Design review of the part built by this model. Coordinates are the model's own, in mm. Face numbers are marked on the shaded views. A direction names the side the tool comes from. Round coordinates to 2 decimals unless told otherwise and drop trailing zeros. Order: outer loops, then holes, each group sorted by start corner. A loop starts at its lowest first (then second) coordinate and runs counter-clockwise, first axis right, second up. Notation, with made-up numbers: (66, 51.25) - (72, 51.25) arc R27 cw to (72, 67.25) - close; hole circle Ø2 at (9, 72). An arc over 180 degrees is marked (long way). Use CSV: the item, a comma, the result in double quotes. Start each with the question number.
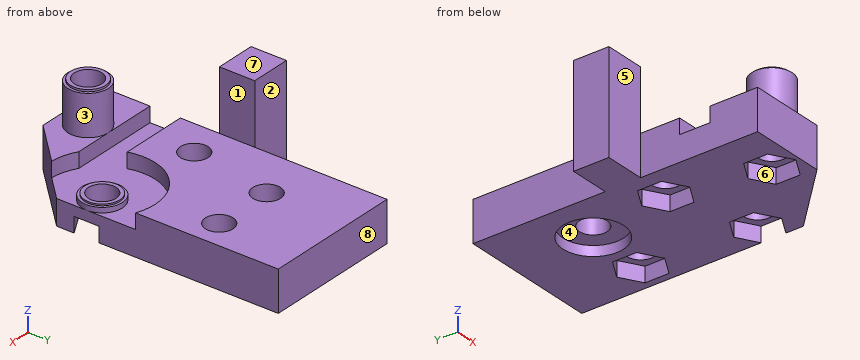
from build123d import *

# Parameters (mm, degrees)
SKETCH007_R             = 2.75
PAD004_DEPTH            = 8
POCKET003_DEPTH         = 3
SKETCH022_R             = 4
SKETCH022_R_2           = 2.75
PAD015_DEPTH            = 1
SKETCH023_R             = 3.5
SKETCH023_R_2           = 2.75
PAD016_DEPTH            = 0.3
SKETCH024_R             = 4
SKETCH024_R_2           = 2.75
PAD017_DEPTH            = 8
SKETCH025_R             = 3.5
SKETCH025_R_2           = 2.75
PAD018_DEPTH            = 0.4
SKETCH026_R             = 6
POCKET005_DEPTH         = 2
POCKET006_DEPTH         = 3
SKETCH028_W             = 7
SKETCH028_H             = 20
PAD019_DEPTH            = 8
BODY001_ROLL_ANGLE      = 180
BODY001_PLACEMENT_ANGLE = -90


with BuildPart() as part:
    # Sketch007 → Pad004 (new body)
    with BuildSketch(Plane.XY):
        Polygon((0, 27.5), (56.4, 27.5), (56.4, 12.5), (43.9, 0), (0, 0), align=None)
        with Locations((16, 17.5)):
            Circle(SKETCH007_R, mode=Mode.SUBTRACT)
        with Locations((16, 5.5)):
            Circle(SKETCH007_R, mode=Mode.SUBTRACT)
        with Locations((32.7, 20.5)):
            Circle(SKETCH007_R, mode=Mode.SUBTRACT)
        with Locations((38, 4)):
            Circle(SKETCH007_R, mode=Mode.SUBTRACT)
        with Locations((50.95, 16.95)):
            Circle(SKETCH007_R, mode=Mode.SUBTRACT)
    extrude(amount=PAD004_DEPTH)

    # Sketch012 (on Face11 of Pad004) → Pocket003 (cut)
    with BuildSketch(Plane(origin=(0, 0, 0), x_dir=(1, 0, 0), z_dir=(0, 0, -1))):
        with BuildLine():
            ThreePointArc((46.95, -9.490674), (31.623381, 4.341986), (40.95, -14.077078))
            Line((40.95, -14.077078), (40.95, -49.490674))
            Line((40.95, -49.490674), (46.95, -49.490674))
            Line((46.95, -9.490674), (46.95, -49.490674))
        make_face()
    extrude(amount=-POCKET003_DEPTH, mode=Mode.SUBTRACT)

    # Sketch022 (on Face2 of Pocket003) → Pad015 (join)
    with BuildSketch(Plane(origin=(0, 0, 3), x_dir=(1, 0, 0), z_dir=(0, 0, -1))):
        with Locations((38, -4)):
            Circle(SKETCH022_R)
        with Locations((38, -4)):
            Circle(SKETCH022_R_2, mode=Mode.SUBTRACT)
    extrude(amount=PAD015_DEPTH)

    # Sketch023 (on Face19 of Pad015) → Pad016 (join)
    with BuildSketch(Plane(origin=(0, 0, 2), x_dir=(1, 0, 0), z_dir=(0, 0, -1))):
        with Locations((38, -4)):
            Circle(SKETCH023_R)
        with Locations((38, -4)):
            Circle(SKETCH023_R_2, mode=Mode.SUBTRACT)
    extrude(amount=PAD016_DEPTH)

    # Sketch024 (on Face18 of Pad016) → Pad017 (join)
    with BuildSketch(Plane(origin=(0, 0, 0), x_dir=(1, 0, 0), z_dir=(0, 0, -1))):
        with Locations((50.95, -16.95)):
            Circle(SKETCH024_R)
        with Locations((50.95, -16.95)):
            Circle(SKETCH024_R_2, mode=Mode.SUBTRACT)
    extrude(amount=PAD017_DEPTH)

    # Sketch025 (on Face23 of Pad017) → Pad018 (join)
    with BuildSketch(Plane(origin=(0, 0, -8), x_dir=(1, 0, 0), z_dir=(0, 0, -1))):
        with Locations((50.95, -16.95)):
            Circle(SKETCH025_R)
        with Locations((50.95, -16.95)):
            Circle(SKETCH025_R_2, mode=Mode.SUBTRACT)
    extrude(amount=PAD018_DEPTH)

    # Sketch026 (on Face6 of Pad018) → Pocket005 (cut)
    with BuildSketch(Plane.XY.offset(8)):
        with Locations((16, 17.5)):
            Circle(SKETCH026_R)
    extrude(amount=-POCKET005_DEPTH, mode=Mode.SUBTRACT)

    # Sketch027 (on Face6 of Pocket005) → Pocket006 (cut)
    with BuildSketch(Plane.XY.offset(8)):
        Polygon((20.75, 5.5), (18.375, 9.613621), (13.625, 9.613621), (11.25, 5.5), (13.625, 1.386379), (18.375, 1.386379), align=None)
        Polygon((37.45, 20.5), (35.075, 24.613621), (30.325, 24.613621), (27.95, 20.5), (30.325, 16.386379), (35.075, 16.386379), align=None)
        Polygon((42.75, 4), (40.375, 8.113621), (35.625, 8.113621), (33.25, 4), (35.625, -0.113621), (40.375, -0.113621), align=None)
        Polygon((55.7, 16.95), (53.325, 21.063621), (48.575, 21.063621), (46.2, 16.95), (48.575, 12.836379), (53.325, 12.836379), align=None)
    extrude(amount=-POCKET006_DEPTH, mode=Mode.SUBTRACT)

    # Sketch028 (on Face12 of Pocket006) → Pad019 (join)
    with BuildSketch(Plane(origin=(0, 27.5, 0), x_dir=(-1, 0, 0), z_dir=(0, 1, 0))):
        with Locations((-29.7, -2)):
            Rectangle(SKETCH028_W, SKETCH028_H)
    extrude(amount=PAD019_DEPTH)


with BuildPart() as part_1:
    # Body001 roll: moved
    add(part.part.rotate(Axis((0, 0, 0), (1, 0, 0)), BODY001_ROLL_ANGLE))


with BuildPart() as part_2:
    # Body001 placement: moved
    add(part_1.part.moved(Location((-37.5, 23, -20))).rotate(Axis((-37.5, 23, -20), (0, 0, 1)), BODY001_PLACEMENT_ANGLE))


solid = part_2.part
Q1. Take a section at D-D (x = -59.5). State the section outline as (y, z) points.
Q2. Take a section at C-C (y = 5.5). State the section outline as (x, z) points, plus the area to 3 significant figures.
Q3. Tool access review of the marked faces 1, 2, 3, 4 and 5: name each direction out of +Z, -Z, +X, -X, +Y, -Y from which nothing blocks a thin tool from reaching the whole face with its end or side.
Q4. For L1, parallel to X at y = 7, z = -23.3; L2, parallel to Y at x = -58, z = -21.75; L3, parallel to Y at x = -43, z = -21.4, list the stretches that pass through material, from the lowest coordinate up. Write a range as [from, to].
Q5. Take a section at A-A (z = -16.5). State the section outline as (x, y) points.
Q6. Take a section at B-B (y = -27.95). State the section outline as (x, z) points.
Q7. Clearance check with flat-ended pins moving along their axes: pin 1 (9 mm diameter, centred on y = 9, z = -25.5, fed in from -X); pin 2 (4 mm diameter, centred on x = -40, y = -16.5, fed in from +Z); pin 3 (3.5 mm diameter, centred on y = -6.5, z = -16, fed in from +X). State where each tip first meets the part, or that it passes through.
Q8. The part is to be moulded in two halves that separate along Y. For the marked faces 6, 7 and 8, say which applies: +Y half, -Y half, draft (parallel to the pull), parting line (faces both ways), or undercut.
Findings below:
1,outline,"(-33.4, -28) - (-13.58, -28) - (-13.58, -25) - (-12, -25) - (-12, -20) - (-17.95, -20) - (-17.95, -23) - (-23.95, -23) - (-23.95, -20) - (-33.4, -20) - close; (-7.4, -25) - (-5.82, -25) - (-5.82, -28) - (3.03, -28) - (3.03, -26) - (10.97, -26) - (10.97, -28) - (23, -28) - (23, -20) - (-7.4, -20) - close"
2,outline,"(-65, -28) - (-60.81, -28) - (-60.81, -26) - (-57.3, -26) - (-57.3, -20) - (-65, -20) - close; (-52.7, -26) - (-49.19, -26) - (-49.19, -28) - (-47.11, -28) - (-47.11, -25) - (-45.3, -25) - (-45.3, -20) - (-52.7, -20) - close; (-40.7, -25) - (-38.89, -25) - (-38.89, -28) - (-37.5, -28) - (-37.5, -20) - (-40.7, -20) - close"
2,area,"121 mm^2"
3,face 1,"+Z, +X, +Y, -Y"
3,face 2,"+Z, -Z, -X, +Y"
3,face 3,"+Z"
3,face 4,"-Z"
3,face 5,"+Z, -Z, -X, -Y"
4,L1,"x = [-65, -57.75], [-52.25, -45.75], [-40.25, -37.5]"
4,L2,"y = [-33.4, -23.95], [-17.95, -12.45], [-6.95, 23]"
4,L3,"y = [-26.4, -25.39], [-4.61, 4.25], [9.75, 23]"
5,outline,"(-73, -10.2) - (-65, -10.2) - (-65, -3.2) - (-73, -3.2) - close; circle Ø8 at (-54.45, -27.95); hole circle Ø5.5 at (-54.45, -27.95)"
6,outline,"(-65, -28) - (-58.56, -28) - (-58.56, -25) - (-57.2, -25) - (-57.2, -11.6) - (-57.95, -11.6) - (-57.95, -12) - (-58.45, -12) - (-58.45, -20) - (-65, -20) - close; (-51.7, -25) - (-50.34, -25) - (-50.34, -28) - (-44.55, -28) - (-44.55, -20) - (-50.45, -20) - (-50.45, -12) - (-50.95, -12) - (-50.95, -11.6) - (-51.7, -11.6) - close"
7,pin 1,"stops at x = -65"
7,pin 2,"stops at z = -21.7"
7,pin 3,"stops at x = -65"
8,face 6,"undercut"
8,face 7,"draft"
8,face 8,"+Y half"
